Autodesk Inventor part; units mm, degrees
ref_plane "YZ Plane" through (0, 0, 0) normal (1, 0, 0) x (0, 1, 0)
ref_plane "XZ Plane" through (0, 0, 0) normal (0, 1, 0) x (-1, 0, 0)
ref_plane "XY Plane" through (0, 0, 0) normal (0, 0, 1) x (1, 0, 0)
sketch "Sketch1" plane through (0, 0, 0) normal (0, 0, 1) x (1, 0, 0)
  line L0 (37.0694, -105.5511) -> (-77.2306, -105.5511)
  line L1 (-77.2306, -105.5511) -> (-77.2306, 123.0489)
  line L2 (-77.2306, 123.0489) -> (37.0694, 123.0489)
  line L3 (37.0694, 123.0489) -> (37.0694, -105.5511)
  line L4 (37.0694, -105.5511) -> (-77.2306, 123.0489) construction
  line L5 (-77.2306, -105.5511) -> (37.0694, 123.0489) construction
  point P0 (0, 0)
  point P1 (-20.0806, 8.7489)
  dimension "d0" = 114.3
  dimension "d1" = 228.6
extrude "Extrusion1" add sketch "Sketch1" along normal blind 6.35
sketch "Sketch2" plane through (0, 0, 6.35) normal (0, 0, 1) x (1, 0, 0)
  line L0 (-77.2306, -105.5511) -> (37.0694, -105.5511)
  line L1 (37.0694, -105.5511) -> (37.0694, 123.0489)
  line L2 (37.0694, 123.0489) -> (-77.2306, 123.0489)
  line L3 (-77.2306, 123.0489) -> (-77.2306, -105.5511)
  circle A0 centre (-33.3319, 108.8699) radius 3.0318
  point P0 (0, 0)
extrude "Extrusion2" add sketch "Sketch2" along normal blind 25.4
properties part number "bottom2 battery holder"
Geometry: final body of the model. Coordinates: model frame, mm. A direction names the side the tool comes from. Round coordinates to 2 decimals unless told otherwise and drop trailing zeros. Use CSV: the item, a comma, the result in double quotes. Start each with the question number.
Q1. Line query: L1, parallel to X at y = 108, z = 14.5; L2, parallel to Y at x = -34, z = 26; L3, parallel to X at y = 107, z = 17. Output: solid intervals per line, ascending.
Q2. First-contact query: pin 1 Ø3 at (x, y) = (-34.5, 108.5) entering from +Z. Flat tip, straight axial feed; report the tip coordinate or a pass-through.
Q3. Reachability of faces 1 (the face through (-21, 10, 31.75)), 2 (the face through (-33, 109, 6.35)) from +Z, -Z, +X, -X, +Y, -Y: full face, straight path, thin tool, end or side. Return the list, or none.
Q4. Pull-direction query (Y, two-part tool) for faces 3 (the face through (-21, 123.049, 16)), 4 (the face through (-19, -105.551, 16)), 5 (the face through (-31.93, 111.56, 18.87)); classes: pulls with the +Y half, pulls with the -Y half, needs draft (parallel to the pull), parting line crosses it, or undercut.
Result sheet:
1,L1,"-77.23 to -36.24, -30.43 to 37.07"
1,L2,"-105.55 to 105.91, 111.83 to 123.05"
1,L3,"-77.23 to -35.72, -30.95 to 37.07"
2,pin 1,"z = 6.35"
3,face 1,"+Z, +X, -X, +Y, -Y"
3,face 2,"+Z"
4,face 3,"pulls with the +Y half"
4,face 4,"pulls with the -Y half"
4,face 5,"undercut"
